```python
from build123d import *

# Parameters (mm, degrees)
F_6_32_TAPPED_HOLE1_REACH  = 74.635
F_6_32_TAPPED_HOLE1_BORE_R = 1.35255
CIRPATTERN2_COUNT          = 4
SKETCH6_R                  = 22.098
SKETCH6_R_2                = 21.7805
BOSS_EXTRUDE1_DEPTH        = 9.906


with BuildPart() as part:
    # Sketch1 → Revolve1 (revolve)
    with BuildSketch(Plane.XY, mode=Mode.PRIVATE) as revolve1_sk:
        Polygon((28.1305, 36.322), (28.1305, 32.512), (23.114, 0), (22.098, 0), (22.098, 32.512), (27.051, 32.512), (27.051, 36.322), align=None)
    revolve(revolve1_sk.sketch.rotate(Axis((0, -2.3241, 0), (0, 1, 0)), 90), axis=Axis((0, -2.3241, 0), (0, 1, 0)))

    # #6-32 Tapped Hole1 bore → #6-32 Tapped Hole1 (cut, up to next)
    with BuildSketch(Plane.XY.offset(28.1305), mode=Mode.PRIVATE) as f_6_32_tapped_hole1_sk1:
        with Locations((0, 22.86)):
            Circle(F_6_32_TAPPED_HOLE1_BORE_R)
    f_6_32_tapped_hole1_tool1 = extrude(f_6_32_tapped_hole1_sk1.sketch, amount=-F_6_32_TAPPED_HOLE1_REACH, mode=Mode.PRIVATE) & part.part
    f_6_32_tapped_hole1 = f_6_32_tapped_hole1_tool1.solids().sort_by_distance((0, 22.86, 28.1305))[0]
    add(f_6_32_tapped_hole1, mode=Mode.SUBTRACT)

    # CirPattern2: #6-32 Tapped Hole1 ×4 about axis
    cirpattern2_axis = Axis((0, 0, 0), (0, 1, 0))
    for i in range(1, CIRPATTERN2_COUNT):
        add(f_6_32_tapped_hole1.rotate(cirpattern2_axis, i * 360 / CIRPATTERN2_COUNT), mode=Mode.SUBTRACT)

    # Sketch6 → Boss-Extrude1 (add)
    with BuildSketch(Plane.XZ):
        with Locations(Location((0, 0, 0), (0, 0, 270))):
            Circle(SKETCH6_R)
        with Locations(Location((0, 0, 0), (0, 0, 270))):
            Circle(SKETCH6_R_2, mode=Mode.SUBTRACT)
    extrude(amount=-BOSS_EXTRUDE1_DEPTH)


solid = part.part
```
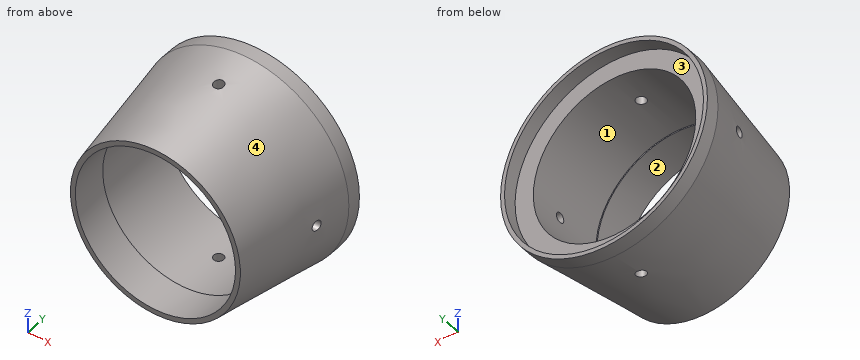
Geometry check sheet. Reference: the model listing, model coordinates, mm. Face numbers are marked on the shaded views. A direction names the side the tool comes from. Coordinates: 2 decimals unless noted, no trailing zeros. Order: outer loops, then holes, each group sorted by start corner. A loop starts at its lowest first (then second) coordinate and runs counter-clockwise, first axis right, second up.
Q1. Sectioned sample at A-A on x = 0. Record the cut outline in (y, z), and give its area (3 significant figures).
Reply:
outline: (0, -23.11) - (21.51, -26.43) - (21.51, -22.1) - (9.91, -22.1) - (9.91, -21.78) - (0, -21.78) - close; (0, 21.78) - (9.91, 21.78) - (9.91, 22.1) - (21.51, 22.1) - (21.51, 26.43) - (0, 23.11) - close; (24.21, -26.85) - (32.51, -28.13) - (36.32, -28.13) - (36.32, -27.05) - (32.51, -27.05) - (32.51, -22.1) - (24.21, -22.1) - close; (24.21, 22.1) - (32.51, 22.1) - (32.51, 27.05) - (36.32, 27.05) - (36.32, 28.13) - (32.51, 28.13) - (24.21, 26.85) - close
area: 219 mm2
Q2. Draft check along Z on the marked faces 3 and 4. Enter one of: released by +Z, released by -Z, zero draft, split by the parting line, or undercut.
Reply:
face 3: undercut
face 4: split by the parting line
Q3. Sectioned sample at D-D on y = 8. Record the cut outline in (x, z), and give its area (3 significant figures).
Reply:
outline: circle Ø48.7 at (0, 0); hole circle Ø43.56 at (0, 0)
area: 372 mm2
Q4. Thickness scan on probe 1 along X at (y, z) = (35.55, 0); probe 2 along Y at (x, z) = (-22, 1); probe 3 along Z at (x, y) = (-2, 31.5). Record the ranges inside material, lowest first.
Reply:
probe 1: x = -28.13 to -27.05, 27.05 to 28.13
probe 2: y = 0 to 9.91
probe 3: z = -27.9 to -22.01, 22.01 to 27.9
Q5. Depth check by flat-ended pin: pin 1 Ø3 at (y, z) = (6, -15.5) entering from -X; pin 2 Ø10 at (y, z) = (30.5, -4.5) entering from -X; pin 3 Ø3 at (y, z) = (30.5, 10) entering from -X. Enter the tip coordinate at first touch or a pass-through.
Reply:
pin 1: stops at x = -19.58
pin 2: stops at x = -28.13
pin 3: stops at x = -26.55
Q6. Tool access check on the marked faces 1 and 2. Record the directions out of +Z, -Z, +X, -X, +Y, -Y that give a thin tool (end or side, any length) a straight path to the whole face; none if there is none.
Reply:
face 1: +Y
face 2: +Y, -Y
Q7. Sectioned sample at B-B on y = 22.86. Record the cut outline in (x, z), and give its area (3 significant figures).
Reply:
outline: (-26.61, -1.35) arc R26.64 ccw to (-1.35, -26.61) - (-1.35, -22.06) arc R22.1 cw to (-22.06, -1.35) - close; (-26.61, 1.35) - (-22.06, 1.35) arc R22.1 cw to (-1.35, 22.06) - (-1.35, 26.61) arc R26.64 ccw to start; (1.35, -26.61) arc R26.64 ccw to (26.61, -1.35) - (22.06, -1.35) arc R22.1 cw to (1.35, -22.06) - close; (1.35, 22.06) arc R22.1 cw to (22.06, 1.35) - (26.61, 1.35) arc R26.64 ccw to (1.35, 26.61) - close
area: 646 mm2
Q8. Sectioned sample at C-C on y = 27.5. Record the cut outline in (x, z), and give its area (3 significant figures).
Reply:
outline: circle Ø54.71 at (0, 0); hole circle Ø44.2 at (0, 0)
area: 817 mm2
